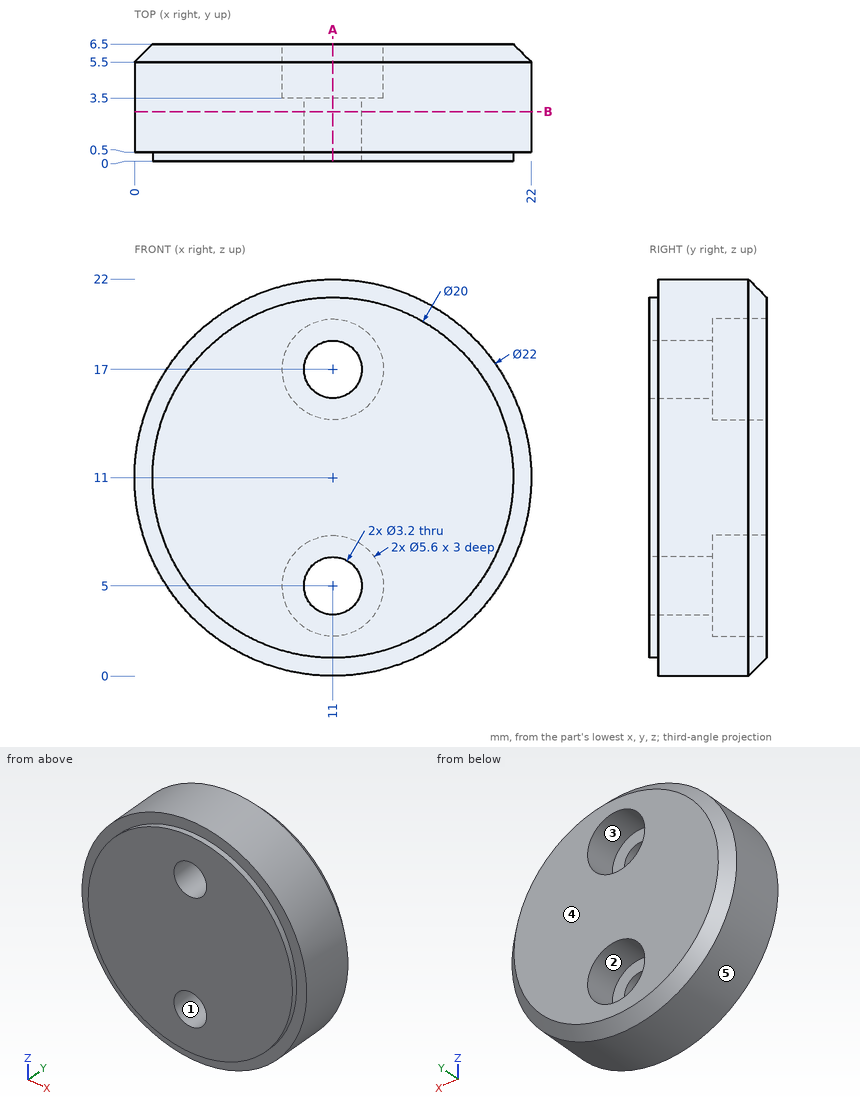
Geometry check sheet. Reference: drawing and pictorial views, mm from the part's lowest x, y, z. A direction names the side the tool comes from. Round coordinates to 2 decimals unless told otherwise and drop trailing zeros. Loops run counter-clockwise (first coordinate to the right, second up) from the corner with the lowest first, then second, coordinate; pieces in that order, holes last. Notation, with made-up numbers: (39, 18.5) - (53, 18.5) arc R26 cw to (53, 55.5) - close; hole circle Ø9 at (4, 58.25). An arc over 180 degrees is marked (long way). Use a Markdown table: item, result.
Q1. Cross-section at A-A on x = 11. Record the cut outline in (y, z), plus the area to 3 significant figures.
Solutions:
| item | result |
|---|---|
| outline | (0, 1) - (0.5, 1) - (0.5, 0) - (5.5, 0) - (6.5, 1) - (6.5, 2.2) - (3.5, 2.2) - (3.5, 3.4) - (0, 3.4) - close; (0, 6.6) - (3.5, 6.6) - (3.5, 7.8) - (6.5, 7.8) - (6.5, 14.2) - (3.5, 14.2) - (3.5, 15.4) - (0, 15.4) - close; (0, 18.6) - (3.5, 18.6) - (3.5, 19.8) - (6.5, 19.8) - (6.5, 21) - (5.5, 22) - (0.5, 22) - (0.5, 21) - (0, 21) - close |
| area | 85.0 mm2 |
Q2. Draft check along Z on the marked faces 3, 4 and 5. Enter one of: released by +Z, released by -Z, zero draft, split by the parting line, or undercut.
Solutions:
| item | result |
|---|---|
| face 3 | undercut |
| face 4 | zero draft |
| face 5 | split by the parting line |
Q3. Access from +Z, -Z, +X, -X, +Y, -Y to the whole of each face (thin tool, end or side, straight path). Record for the marked faces 1 and 2.
Solutions:
| item | result |
|---|---|
| face 1 | +Y, -Y |
| face 2 | +Y |
Q4. Cross-section at B-B on y = 2.75. Record the cut outline in (x, z).
Solutions:
| item | result |
|---|---|
| outline | circle Ø22 at (11, 11); hole circle Ø3.2 at (11, 5); hole circle Ø3.2 at (11, 17) |
Q5. Material ranges on line 1 (Z direction, x = 9, y = 3.75); line 2 (X direction, y = 1.3, z = 17); line 3 (X direction, y = 2.5, z = 6), recorded low to high.
Solutions:
| item | result |
|---|---|
| line 1 | z = 0.18 to 3.04, 6.96 to 15.04, 18.96 to 21.82 |
| line 2 | x = 1.78 to 9.4, 12.6 to 20.22 |
| line 3 | x = 1.2 to 9.75, 12.25 to 20.8 |
Q6. Go/stop test with flat-tipped pins: P1, Ø1, axis at x = 13.5, y = 1, coming from the -Z side; P2, Ø1.7, axis at x = 11, z = 16, coming from the +Y side; P3, Ø1.9, axis at x = 11, z = 17, coming from the -Y side. Record where each tip stops, or that it passes through.
Solutions:
| item | result |
|---|---|
| P1 | stops at z = 0.18 |
| P2 | stops at y = 3.5 |
| P3 | passes through |
